The listing builds one solid part. Answer for the finished solid, in the listing's coordinates (mm). A direction names the side the tool comes from. Give positions to 0.01 mm unless a question says otherwise; leave off trailing zeros. Loops run counter-clockwise (first coordinate to the right, second up) from the corner with the lowest first, then second, coordinate; pieces in that order, holes last. Notation, with made-up numbers: M 3,-27.5 L 55,-27.5 A26 ccw 55,5.5 Z; hole C -36.75,-26 d8. An arc over 180 degrees is marked long. One line per item, written item: value. Start each with the question number.
Q1. Consider L1, parallel to X at y = 25, z = 35; L2, parallel to X at y = 1.5, z = 40; L3, parallel to Y at x = 39, z = 10.5. Determine where each line is inside the solid, lowest interval first.
Q2. A cutting plane is placed at B-B, the plane x = 15. Determine the outline of the cut face in (y, z), and give its area (3 significant figures).
Q3. The mould has two halves that part along Y. Classify faces 1 (the cylindrical face through (55.21, 0.88, 39.99)), 2 (the cylindrical face through (-55.14, 0.92, 41.99)), 3 (the flat face through (45, 8, 42)), 4 (the cylindrical face through (-67.465, 17.589, 43.234)): +Y half, -Y half, draft (parallel to the pull), parting line (faces both ways), or undercut.
Q4. A cutting plane is placed at A-A, the plane x = -52.5. Determine the outline of the cut face in (y, z), and give its area (3 significant figures).
Q5. For faces 5 (the flat face through (-45, -8, 42)), 6 (the flat face through (-0.3, 49.5, 0)), 7 (the cylindrical face through (-67.46, 40.07, 18.01)), 8 (the flat face through (-70, 7, 40)), 9 (the cylindrical face through (67.465, -17.147, 43.273)), determine the directions among +Z, -Z, +X, -X, +Y, -Y from which every point of the face is accessible in a straight line to the end or side of a thin tool.
Q6. Flat-ended cylindrical pins translate along their axes: pin 1 (2 mm diameter, centred on x = 18.5, z = 12.5, fed in from +Y); pin 2 (3 mm diameter, centred on x = 20, y = -23.5, fed in from -Z); pin 3 (8 mm diameter, centred on x = -1.5, z = 33, fed in from +Y); pin 4 (4.5 mm diameter, centred on y = 17.22, z = 41.57, fed in from +X). Find the tip coordinate at first contact, or state that the pin passes through.
from build123d import *

# Parameters (mm, degrees)
REVOLVE_1_ANGLE          = 180
HOLE_WIZARD_M3_1_D       = 3.4
HOLE_WIZARD_M3_1_DEPTH   = 5
PATTERN_CIRCULAR_1_COUNT = 4
PATTERN_CIRCULAR_1_ANGLE = 135
MIRROR_1_COPY_1_D        = 3.4
MIRROR_1_COPY_1_DEPTH    = 5
MIRROR_1_COPY_2_D        = 3.4
MIRROR_1_COPY_2_DEPTH    = 5
MIRROR_1_COPY_3_D        = 3.4
MIRROR_1_COPY_3_DEPTH    = 5
FILLET_1_R               = 9


with BuildPart() as part:
    # ｽｹｯﾁ1 → 回転1 (revolve)
    with BuildSketch(Plane.XY):
        Polygon((-70, 40), (-40, 40), (-40, 49), (40, 49), (40, 40), (70, 40), (70, 50), (65, 50), (65, 42), (45, 42), (45, 50), (-45, 50), (-45, 42), (-65, 42), (-65, 50), (-70, 50), align=None)
    revolve(axis=Axis((-50, 0, 0), (1, 0, 0)), revolution_arc=REVOLVE_1_ANGLE)

    # M3 すきま穴1
    with Locations(Plane.ZY.offset(70)):
        with Locations((17.220754456, -41.574578963)):
            hole_wizard_m3_1 = Hole(HOLE_WIZARD_M3_1_D / 2, depth=HOLE_WIZARD_M3_1_DEPTH)

    # 円形ﾊﾟﾀｰﾝ1: M3 すきま穴1 ×4 about axis
    pattern_circular_1_axis = Axis((0, 0, 0), (-1, 0, 0))
    for i in range(1, PATTERN_CIRCULAR_1_COUNT):
        add(hole_wizard_m3_1.rotate(pattern_circular_1_axis, i * PATTERN_CIRCULAR_1_ANGLE / (PATTERN_CIRCULAR_1_COUNT - 1)), mode=Mode.SUBTRACT)

    # ﾐﾗｰ1: M3 すきま穴1 across plane
    add(hole_wizard_m3_1.mirror(Plane(origin=(0, 0, 0), x_dir=(0, 0, 1), z_dir=(1, 0, 0))), mode=Mode.SUBTRACT)

    # ﾐﾗｰ1 copy 1
    with Locations(Plane(origin=(70, 0, 0), x_dir=(0, 0.7071067811865487, 0.7071067811865464), z_dir=(1, 0, 0))):
        with Locations((17.220754456, 41.574578963)):
            Hole(MIRROR_1_COPY_1_D / 2, depth=MIRROR_1_COPY_1_DEPTH)

    # ﾐﾗｰ1 copy 2
    with Locations(Plane.YZ.offset(70)):
        with Locations((17.220754456, 41.574578963)):
            Hole(MIRROR_1_COPY_2_D / 2, depth=MIRROR_1_COPY_2_DEPTH)

    # ﾐﾗｰ1 copy 3
    with Locations(Plane(origin=(70, 0, 0), x_dir=(0, 0.7071067811865441, -0.7071067811865509), z_dir=(1, 0, 0))):
        with Locations((17.220754456, 41.574578963)):
            Hole(MIRROR_1_COPY_3_D / 2, depth=MIRROR_1_COPY_3_DEPTH)

    # ﾌｨﾚｯﾄ1
    fillet_1_edges = [part.edges().sort_by_distance(p)[0] for p in [
        (-40, 0, 49),
        (40, 0, 49),
    ]]
    fillet(fillet_1_edges, radius=FILLET_1_R - 0.0001)  # a hair under: the kernel refuses the full size


solid = part.part
Answer block:
1. L1: -70 to -65, -45 to -39.48, 39.48 to 45, 65 to 70
1. L2: -70 to -40, 40 to 70
1. L3: -48.89 to -42.86, 42.86 to 48.89
2. outline: M -50,0 L -49,0 A49 cw 49,0 L 50,0 A50 ccw Z
2. area: 156 mm^2
3. face 1: undercut
3. face 2: parting line
3. face 3: draft
3. face 4: undercut
4. outline: M -42,0 L -40,0 A40 cw 40,0 L 42,0 A42 ccw Z
4. area: 258 mm^2
5. face 5: +Z
5. face 6: -Z, +X, -X, +Y, -Y
5. face 7: -X
5. face 8: +Z, -Z, -X, +Y, -Y
5. face 9: +X
6. pin 1: y = 48.66
6. pin 2: z = 42.14
6. pin 3: y = 40.73
6. pin 4: x = 70
